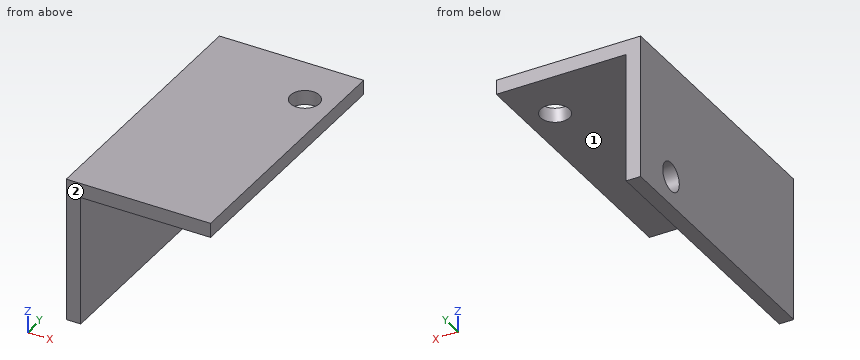
```python
from build123d import *

# Parameters (mm, degrees)
BOSS_EXTRUDE1_DEPTH = 21
SKETCH2_R           = 1
CUT_EXTRUDE1_DEPTH  = 21
CUT_EXTRUDE2_DEPTH  = 2.48
SKETCH4_R           = 1
CUT_EXTRUDE3_DEPTH  = 2.48


with BuildPart() as part:
    # Sketch1 → Boss-Extrude1 (new body)
    with BuildSketch(Plane(origin=(0, 0, 0), x_dir=(1, 0, 0), z_dir=(0, 1, 0))):
        Polygon((0, 0), (0, 10), (1, 10), (1, 1), (10, 1), (10, 0), align=None)
    extrude(amount=BOSS_EXTRUDE1_DEPTH)

    # Sketch2 → Cut-Extrude1 (cut)
    with BuildSketch(Plane(origin=(0, 0, -1), x_dir=(-1, 0, 0), z_dir=(0, 0, -1))):
        with Locations((-8, 17.381971211)):
            Circle(SKETCH2_R)
    extrude(amount=-CUT_EXTRUDE1_DEPTH, mode=Mode.SUBTRACT)

    # Sketch3 → Cut-Extrude2 (cut)
    with BuildSketch(Plane.XZ):
        Polygon((10, 0), (10, -1), (1, -1), (1, -10), (0, -10), (0, 0), align=None)
    extrude(amount=-CUT_EXTRUDE2_DEPTH, mode=Mode.SUBTRACT)

    # Sketch4 → Cut-Extrude3 (cut)
    with BuildSketch(Plane(origin=(1, 0, 0), x_dir=(0, 0, -1), z_dir=(1, 0, 0))):
        with Locations((8, 17.32)):
            Circle(SKETCH4_R)
    extrude(amount=-CUT_EXTRUDE3_DEPTH, mode=Mode.SUBTRACT)


solid = part.part
```
The model under review builds one solid part; all positions refer to its coordinate system, in mm. Face numbers are marked on the shaded views. A direction names the side the tool comes from. Give positions to 0.01 mm unless a question says otherwise; leave off trailing zeros. Order: outer loops, then holes, each group sorted by start corner. A loop starts at its lowest first (then second) coordinate and runs counter-clockwise, first axis right, second up. Notation, with made-up numbers: (63.25, 28.25) - (117.25, 28.25) arc R8 cw to (117.25, 33.25) - close; hole circle Ø7 at (6, 46.5). An arc over 180 degrees is marked (long way). Use CSV: the item, a comma, the result in double quotes. Start each with the question number.
Q1. We need section D-D, the plane z = -5.25. Write out the cut boundary in (x, y).
Q2. To check wall thickness, follow line 1 along Y through (x, z) = (8, -0.7); line 2 along Y through (x, z) = (0.8, -8); line 3 along Z through (x, y) = (4, 17.25). State the ranges of each line that lie inside material, in increasing order. Write a range as [from, to].
Q3. We need section C-C, the plane y = 10. Write out the cut boundary in (x, z).
Q4. We need section A-A, the plane z = -8. Write out the cut boundary in (x, y), and give its area (3 significant figures).
Q5. Clearance check with flat-ended pins moving along their axes: pin 1 Ø5 at (y, z) = (8, -4) entering from +X; pin 2 Ø2.5 at (x, y) = (6, 14.5) entering from -Z; pin 3 Ø1.2 at (x, y) = (8, 17.38) entering from +Z. State where each tip first meets the part, or that it passes through.
Q6. We need section B-B, the plane x = 8.5. Write out the cut boundary in (y, z).
Q7. Tool access review of the marked faces 1 and 2: name each direction out of +Z, -Z, +X, -X, +Y, -Y from which nothing blocks a thin tool from reaching the whole face with its end or side.
Outcome:
1,outline,"(0, 2.48) - (1, 2.48) - (1, 21) - (0, 21) - close"
2,line 1,"y = [2.48, 16.38], [18.38, 21]"
2,line 2,"y = [2.48, 16.32], [18.32, 21]"
2,line 3,"z = [-1, 0]"
3,outline,"(0, -10) - (1, -10) - (1, -1) - (10, -1) - (10, 0) - (0, 0) - close"
4,outline,"(0, 2.48) - (1, 2.48) - (1, 16.32) - (0, 16.32) - close; (0, 18.32) - (1, 18.32) - (1, 21) - (0, 21) - close"
4,area,"16.5 mm^2"
5,pin 1,"stops at x = 1"
5,pin 2,"stops at z = -1"
5,pin 3,"passes through"
6,outline,"(2.48, -1) - (16.52, -1) - (16.52, 0) - (2.48, 0) - close; (18.25, -1) - (21, -1) - (21, 0) - (18.25, 0) - close"
7,face 1,"-Z, +X, +Y, -Y"
7,face 2,"+Z, -Z, +X, -X, -Y"
